Can you work these out from the model? Positions are in its coordinate system, mm. Give positions to 0.01 mm unless a question says otherwise; leave off trailing zeros. Write each loop counter-clockwise with the first axis right and the second up, starting at its lowest first coordinate (ties: lowest second). Pieces come first, ordered by that corner, then holes.
1. Suppose I cut it at B-B (x = 181.5). Please give me the cut outline in (y, z), and give its area (3 significant figures).
2. I'm going to push flat-ended pins straight in: pin 1 (2 mm diameter, centred on y = -332.5, z = 3.5, fed in from -X); pin 2 (1.5 mm diameter, centred on y = -412, z = 14, fed in from -X); pin 3 (10 mm diameter, centred on y = -318, z = 3.5, fed in from +X). Where does each tip first touch, or does it pass through?
3. If I drill on probe 1 along Y at (x, z) = (154.5, -10); probe 2 along Y at (x, z) = (40.5, 2); probe 3 along X at (y, z) = (-323, -14), over which ranges is the centre line in solid material (lowest first)?
4. Suppose I cut it at A-A (z = -11.5). Please give me the cut outline in (x, y), and give its area (3 significant figures).
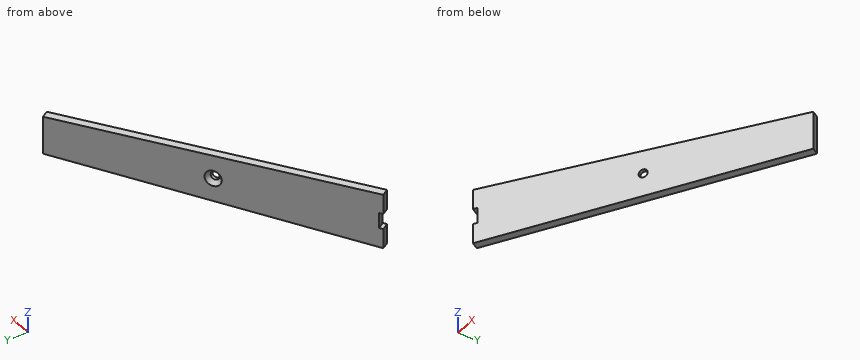
Autodesk Inventor part; units mm, degrees
ref_plane "Work Plane1" through (216.1794, 0, 0) normal (1, 0, 0) x (0, 1, 0)
ref_plane "Work Plane2" through (0, -431.2082, -22.5987) normal (-0.5244795, 0.8514231, 0) x (0, 0, 1)
ref_plane "XZ Plane" through (0, 0, 0) normal (0, 1, 0) x (-1, 0, 0)
sketch "Sketch1" plane through (0, 0, 0) normal (1, 0, 0) x (0, 1, 0)
  circle A0 centre (0, 0) radius 431.8 construction
  line L0 (-431.2082, -22.5987) -> (-431.2082, 22.5987)
  line L1 (-431.2082, -22.5987) -> (-386.0109, -22.5987) construction
  line L2 (-431.2082, -22.5987) -> (0, 0) construction
  line L3 (0, 0) -> (-431.2082, 22.5987) construction
  dimension "d0" = 863.6
  dimension "d3" = 90
  dimension "d4" = 6
ref_plane "Work Plane1" through (216.1794, 0, 0) normal (1, 0, 0) x (0, 1, 0)
sketch "Sketch2" plane through (216.1794, 0, 0) normal (1, 0, 0) x (0, 1, 0)
  circle A0 centre (0, 0) radius 298.45 construction
  line L0 (-298.041, 15.6197) -> (-298.041, -15.6197)
  line L1 (-298.041, 15.6197) -> (-266.8017, 15.6197) construction
  line L2 (-298.041, 15.6197) -> (0, 0) construction
  line L3 (0, 0) -> (-298.041, -15.6197) construction
  dimension "d2" = 596.9
  dimension "d5" = 90
  dimension "d6" = 6
ref_plane "Work Plane2" through (0, -431.2082, -22.5987) normal (-0.5244795, 0.8514231, 0) x (0, 0, 1)
sketch "Sketch3" plane through (0, -431.2082, -22.5987) normal (-0.5244795, 0.8514231, 0) x (0, 0, 1)
  line L0 (0, 0) -> (45.1973, 0)
  line L1 (38.2183, 253.9036) -> (6.979, 253.9036)
  line L2 (6.979, 253.9036) -> (0, 0)
  line L3 (45.1973, 0) -> (38.2183, 253.9036)
  point P0 (22.5987, 226.1599)
extrude "Extrusion1" add sketch "Sketch3" against normal blind 6.35
sketch "Sketch5" plane through (0, -431.2082, -22.5987) normal (-0.5244795, 0.8514231, 0) x (0.8514231, 0.5244795, 0)
  line L0 (-3.175, -28.9487) -> (3.175, -28.9487)
  line L1 (3.175, -28.9487) -> (3.175, -16.2487)
  line L2 (3.175, -16.2487) -> (-3.175, -16.2487)
  line L3 (-3.175, -16.2487) -> (-3.175, -28.9487)
  line L4 (0, -45.1973) -> (0, 0)
  line L5 (-3.175, -28.9487) -> (3.175, -16.2487) construction
  line L6 (3.175, -28.9487) -> (-3.175, -16.2487) construction
  point P0 (226.1599, -22.5987)
  point P1 (0, -22.5987)
  point P2 (0, -28.9487)
  point P3 (0, -16.2487)
  dimension "d17" = 6.35
  dimension "d18" = 12.7
extrude "Extrusion3" cut sketch "Sketch5" against normal through all
sketch "Sketch6" plane through (0, -431.2082, -22.5987) normal (-0.5244795, 0.8514231, 0) x (0.8514231, 0.5244795, 0)
  line L0 (253.9036, -38.2183) -> (253.9036, -6.979)
  line L1 (0, 0) -> (0, -16.2487)
  line L2 (253.9036, -6.979) -> (253.9036, -38.2183)
  line L3 (253.9036, -22.5987) -> (3.175, -22.5987) construction
  line L4 (3.175, -16.2487) -> (3.175, -28.9487)
  point P0 (226.1599, -22.5987)
  point P1 (126.9518, -22.5987)
  dimension "d21" = 253.9036
  dimension "d22" = 126.9518
hole "Hole1" at (108.0897, -364.6246, 0) direction (0.5244795, -0.8514231, 0) diameter 6.7564 end through all countersink diameter 12.8778 countersink angle 82
properties part number "Touch Fifth" material "Polycarbonate, Clear"
Checks:
1. outline: (-326.86, -16.85) - (-319.4, -16.74) - (-319.4, 16.74) - (-326.86, 16.85) - close
1. area: 250 mm2
2. pin 1: stops at x = 158.62
2. pin 2: stops at x = 29.96
2. pin 3: stops at x = 204
3. probe 1: y = -343.49 to -336.04
3. probe 2: y = -413.72 to -406.26
3. probe 3: x = 175.66 to 187.77
4. outline: (0, -431.21) - (3.33, -436.61) - (219.51, -303.45) - (216.18, -298.04) - close
4. area: 1,610 mm2
